Geometry: final body of the model. Coordinates: model frame, mm. A direction names the side the tool comes from. Coordinates: 2 decimals unless noted, no trailing zeros. Order: outer loops, then holes, each group sorted by start corner. A loop starts at its lowest first (then second) coordinate and runs counter-clockwise, first axis right, second up. Notation, with made-up numbers: (35.25, 25.5) - (94.25, 25.5) arc R15 ccw to (94.25, 52.5) - close; hole circle Ø7 at (1.25, -24.75). An arc over 180 degrees is marked (long way). Use a Markdown table: item, result. Add a question column.
```python
from build123d import *

# Parameters (mm, degrees)
SKETCH1_R           = 4
BOSS_EXTRUDE1_DEPTH = 220
SKETCH2_R           = 3.125
CUT_EXTRUDE1_DEPTH  = 6.5


with BuildPart() as part:
    # Sketch1 → Boss-Extrude1 (new body)
    with BuildSketch(Plane.XY):
        Circle(SKETCH1_R)
    extrude(amount=BOSS_EXTRUDE1_DEPTH)

    # Sketch2 → Cut-Extrude1 (cut)
    with BuildSketch(Plane.XY.offset(220)):
        Circle(SKETCH2_R)
    cut_extrude1 = extrude(amount=-CUT_EXTRUDE1_DEPTH, mode=Mode.SUBTRACT)

    # Mirror1: Cut-Extrude1 across plane
    add(cut_extrude1.mirror(Plane.XY.offset(110)), mode=Mode.SUBTRACT)


solid = part.part
```
1) Set-up query: faces 5 (the face through (0, 0, 6.5)), 6 (the face through (2, -3, 0)). Return all of +Z, -Z, +X, -X, +Y, -Y with unobstructed straight access to the full face (end or side cutting, diameter ignored); none if empty.
2) Draft query along X for faces 1 (the face through (0, 0, 213.5)), 2 (the face through (2.98, 0.94, 216.8)), 3 (the face through (2, -3, 220)), 4 (the face through (-0.867, -3.905, 108.46)). Return one class per face: pulls with the +X half, pulls with the -X half, needs draft (parallel to the pull), parting line crosses it, or undercut.
3) Section A-A (x = 0). Return loops of the section in (y, z) (3 decimals), then the cut area to 3 significant figures.
4) Pin query (flat end, axial travel): pin 1 (3 mm diameter, centred on x = 0.5, y = -0.5, fed in from +Z); pin 2 (2 mm diameter, centred on x = -0.5, y = -1.5, fed in from -Z); pin 3 (1.5 mm diameter, centred on y = 2, z = 173.5, fed in from -X). Return the tip coordinate at first contact, or that it passes through.
5) Ray query, line 1 along Y through (x, z) = (0, 218.25) (3 decimals); line 2 along Z through (x, y) = (1.75, -0.5); line 3 along X through (y, z) = (-0.5, 17). Return the intervals inside material, ascending.
6) Section C-C (z = 24). Return loops of the section in (x, y), then the cut area to 3 significant figures.
Values follow:
| question | item | result |
|---|---|---|
| 1 | face 5 | -Z |
| 1 | face 6 | -Z, +X, -X, +Y, -Y |
| 2 | face 1 | undercut |
| 2 | face 2 | undercut |
| 2 | face 3 | needs draft |
| 2 | face 4 | parting line crosses it |
| 3 | outline | (-4, 0) - (-3.125, 0) - (-3.125, 6.5) - (3.125, 6.5) - (3.125, 0) - (4, 0) - (4, 220) - (3.125, 220) - (3.125, 213.5) - (-3.125, 213.5) - (-3.125, 220) - (-4, 220) - close |
| 3 | area | 1,680 mm² |
| 4 | pin 1 | stops at z = 213.5 |
| 4 | pin 2 | stops at z = 6.5 |
| 4 | pin 3 | stops at x = -3.8 |
| 5 | line 1 | y = -4 to -3.125, 3.125 to 4 |
| 5 | line 2 | z = 6.5 to 213.5 |
| 5 | line 3 | x = -3.97 to 3.97 |
| 6 | outline | circle Ø8 at (0, 0) |
| 6 | area | 50.3 mm² |
